The listing builds one solid part. Answer for the finished solid, in the listing's coordinates (mm). A direction names the side the tool comes from. Round coordinates to 2 decimals unless told otherwise and drop trailing zeros. Order: outer loops, then holes, each group sorted by start corner. A loop starts at its lowest first (then second) coordinate and runs counter-clockwise, first axis right, second up. Notation, with made-up numbers: (-10, 24.25) -> (43, 24.25) arc R27 ccw to (43, 58.25) -> close; hole circle Ø6 at (12.5, 64). An arc over 180 degrees is marked (long way). Answer in a Markdown table with one row per item. Add a question column.
Autodesk Inventor part; units mm, degrees
ref_plane "YZ Plane" through (0, 0, 0) normal (1, 0, 0) x (0, 1, 0)
ref_plane "XZ Plane" through (0, 0, 0) normal (0, 1, 0) x (-1, 0, 0)
ref_plane "XY Plane" through (0, 0, 0) normal (0, 0, 1) x (1, 0, 0)
sketch "Boceto1" plane through (0, 0, 0) normal (0, 1, 0) x (-1, 0, 0)
  line L0 (0, 0) -> (-1850, 0)
  line L1 (-1850, 0) -> (-1850, -720)
  line L2 (-1850, -720) -> (0, -720)
  line L3 (0, -720) -> (0, 0)
  dimension "d0" = 1850
  dimension "d1" = 720
extrude "Extrusión1" add sketch "Boceto1" along normal blind 700
sketch "Boceto2" plane through (0, 0, 0) normal (0, -1, 0) x (1, 0, 0)
  line L0 (1850, 0) -> (1850, -720)
  line L1 (0, 0) -> (1850, 0)
  line L2 (0, -720) -> (0, 0)
  line L3 (1850, -720) -> (0, -720)
  line L4 (140, -580) -> (140, -140)
  line L5 (1710, -140) -> (1710, -580)
  line L6 (1710, -580) -> (140, -580)
  line L7 (1710, -140) -> (1710, 0)
  line L8 (140, -140) -> (140, 0)
  dimension "d4" = 140
extrude "Extrusión2" cut sketch "Boceto2" against normal blind 350 contours L7 L5 L6 L4 L8 L1
properties part number "sofa"
1. Each of these flat-tipped pins is pushed along its axis until it touches: pin 1 (10 mm diameter, centred on x = 1385, y = 602.5, fed in from +Z); pin 2 (2 mm diameter, centred on x = 1165.5, z = -148.5, fed in from -Y). Where does it stop, or does it pass through?
2. The part is cut by section B-B (x = 1433.5). Give the vertices of the cut face in (y, z).
3. For faces 1 (the flat face through (914, 350, -286)), 2 (the flat face through (938, 700, -355)), determine the directions among +Z, -Z, +X, -X, +Y, -Y from which every point of the face is accessible in a straight line to the end or side of a thin tool.
4. The part is cut by section A-A (z = -107). Give the vertices of the cut face in (x, y).
5. The part is cut by section C-C (y = 196). Give the vertices of the cut face in (x, z), then the cut area to 3 significant figures.
6. Straight lines are drawn through the part: line 1 along X through (y, z) = (122, -39); line 2 along Y through (x, z) = (766, -442.5); line 3 along Z through (x, y) = (1201, 332). For each, find the intervals that lie inside material, in ascending order.
Report:
| question | item | result |
|---|---|---|
| 1 | pin 1 | stops at z = 0 |
| 1 | pin 2 | stops at y = 350 |
| 2 | outline | (0, -720) -> (700, -720) -> (700, 0) -> (350, 0) -> (350, -580) -> (0, -580) -> close |
| 3 | face 1 | +Z, -Y |
| 3 | face 2 | +Z, -Z, +X, -X, +Y |
| 4 | outline | (0, 0) -> (140, 0) -> (140, 350) -> (1710, 350) -> (1710, 0) -> (1850, 0) -> (1850, 700) -> (0, 700) -> close |
| 5 | outline | (0, -720) -> (1850, -720) -> (1850, 0) -> (1710, 0) -> (1710, -580) -> (140, -580) -> (140, 0) -> (0, 0) -> close |
| 5 | area | 421,000 mm^2 |
| 6 | line 1 | x = 0 to 140, 1710 to 1850 |
| 6 | line 2 | y = 350 to 700 |
| 6 | line 3 | z = -720 to -580 |
